Read the model definition and answer for the solid it produces. Units are mm, in the model's axes. Face numbers are marked on the shaded views. A direction names the side the tool comes from. Round coordinates to 2 decimals unless told otherwise and drop trailing zeros. Loops run counter-clockwise (first coordinate to the right, second up) from the corner with the lowest first, then second, coordinate; pieces in that order, holes last. Notation, with made-up numbers: (42.5, 31) - (53.5, 31) arc R16 ccw to (53.5, 59) - close; hole circle Ø10 at (82, 72). An arc over 180 degrees is marked (long way). Use one line per item in the form item = value. Start each with the question number.
```python
from build123d import *

# Parameters (mm, degrees)
SKETCH_R     = 12
PAD_DEPTH    = 30
PAD001_DEPTH = 30


with BuildPart() as part:
    # Sketch → Pad (new body)
    with BuildSketch(Plane.XY):
        with BuildLine():
            Line((29.808627, -133.970841), (29.808627, -73.970841))
            Line((29.808627, -73.970841), (-30.191373, -73.970841))
            Line((-30.191373, -73.970841), (-30.191373, -133.970841))
            Line((-59.898036, -134.146891), (-30.191373, -133.970841))
            ThreePointArc((-79.943921, -113.552778), (-74.10502, -127.922494), (-59.898036, -134.146891))
            Line((-79.943921, 100.605318), (-79.943921, -113.552778))
            ThreePointArc((-59.685634, 120.863606), (-74.010406, 114.930091), (-79.943921, 100.605318))
            Line((60.081005, 120.863606), (-59.685634, 120.863606))
            ThreePointArc((80.068853, 100.875757), (74.214548, 115.009301), (60.081005, 120.863606))
            Line((80.068853, -113.591927), (80.068853, 100.875757))
            ThreePointArc((59.515305, -134.144193), (74.048781, -128.125027), (80.068853, -113.591927))
            Line((29.808627, -133.970841), (59.515305, -134.144193))
        make_face()
        with Locations((0.120778, 29.919195)):
            Circle(SKETCH_R, mode=Mode.SUBTRACT)
        with Locations((-53.325886, -24.171413)):
            Circle(SKETCH_R, mode=Mode.SUBTRACT)
        with Locations((55.271923, 86.295181)):
            Circle(SKETCH_R, mode=Mode.SUBTRACT)
    extrude(amount=PAD_DEPTH)

    # Sketch → Pad001 (join)
    with BuildSketch(Plane.XY):
        with BuildLine():
            Line((29.808627, -133.970841), (29.808627, -73.970841))
            Line((29.808627, -73.970841), (-30.191373, -73.970841))
            Line((-30.191373, -73.970841), (-30.191373, -133.970841))
            Line((-59.898036, -134.146891), (-30.191373, -133.970841))
            ThreePointArc((-79.943921, -113.552778), (-74.10502, -127.922494), (-59.898036, -134.146891))
            Line((-79.943921, 100.605318), (-79.943921, -113.552778))
            ThreePointArc((-59.685634, 120.863606), (-74.010406, 114.930091), (-79.943921, 100.605318))
            Line((60.081005, 120.863606), (-59.685634, 120.863606))
            ThreePointArc((80.068853, 100.875757), (74.214548, 115.009301), (60.081005, 120.863606))
            Line((80.068853, -113.591927), (80.068853, 100.875757))
            ThreePointArc((59.515305, -134.144193), (74.048781, -128.125027), (80.068853, -113.591927))
            Line((29.808627, -133.970841), (59.515305, -134.144193))
        make_face()
        with Locations((0.120778, 29.919195)):
            Circle(SKETCH_R, mode=Mode.SUBTRACT)
        with Locations((-53.325886, -24.171413)):
            Circle(SKETCH_R, mode=Mode.SUBTRACT)
        with Locations((55.271923, 86.295181)):
            Circle(SKETCH_R, mode=Mode.SUBTRACT)
    extrude(amount=PAD001_DEPTH)


solid = part.part
```
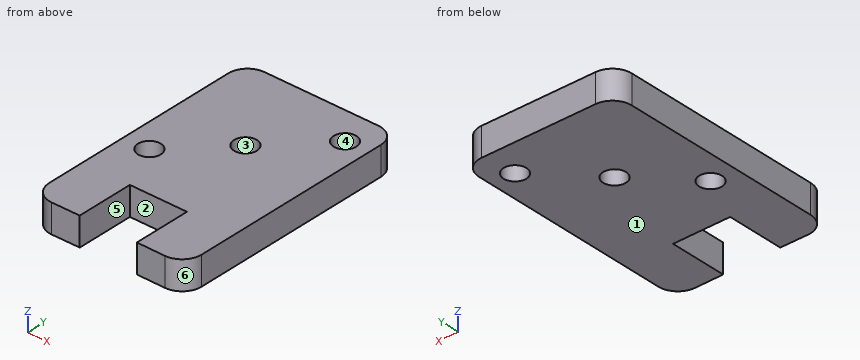
1) Flat-ended cylindrical pins translate along their axes: pin 1 (21.5 mm diameter, centred on x = 0.12, y = 29.92, fed in from -Z); pin 2 (8 mm diameter, centred on x = 51, z = 8.5, fed in from -Y). Find the tip coordinate at first contact, or state that the pin passes through.
2) A cutting plane is placed at B-B on x = 52. Write down the section's boundary in (y, z).
3) A cutting plane is placed at A-A on y = -109. Write down the section's boundary in (x, z).
4) Determine the mould class of the marked faces 1, 2, 3 and 4 for opening direction Y: +Y half, -Y half, draft (parallel to the pull), parting line (faces both ways), or undercut.
5) A cutting plane is placed at C-C on z = 22.5. Write down the section's boundary in (x, y), plus the area to 3 significant figures.
6) A cutting plane is placed at D-D on x = 20. Write down the section's boundary in (y, z), plus the area to 3 significant figures.
7) Straight lines are drawn through the part: line 1 (X direction, y = -95.5, z = 3); line 2 (Y direction, x = -36.5, z = 20.25); line 3 (X direction, y = 95, z = 22.5). For each, find the intervals that lie inside material, in ascending order. Write a range as from..to.
8) For the marked faces 5 and 6, determine the directions among +Z, -Z, +X, -X, +Y, -Y from which every point of the face is accessible in a straight line to the end or side of a thin tool.
Checks:
q1.pin_1 = through
q1.pin_2 = -134.12
q2.outline = (-134.1, 0) - (74.75, 0) - (74.75, 30) - (-134.1, 30) - close; (97.84, 0) - (120.86, 0) - (120.86, 30) - (97.84, 30) - close
q3.outline = (-79.94, 0) - (-30.19, 0) - (-30.19, 30) - (-79.94, 30) - close; (29.81, 0) - (80.07, 0) - (80.07, 30) - (29.81, 30) - close
q4.face_1 = draft
q4.face_2 = -Y half
q4.face_3 = undercut
q4.face_4 = undercut
q5.outline = (-79.94, -113.55) arc R20.6 ccw to (-59.9, -134.15) - (-30.19, -133.97) - (-30.19, -73.97) - (29.81, -73.97) - (29.81, -133.97) - (59.52, -134.14) arc R20.55 ccw to (80.07, -113.59) - (80.07, 100.88) arc R19.99 ccw to (60.08, 120.86) - (-59.69, 120.86) arc R20.26 ccw to (-79.94, 100.61) - close; hole circle Ø24 at (-53.33, -24.17); hole circle Ø24 at (0.12, 29.92); hole circle Ø24 at (55.27, 86.3)
q5.area = 35,500 mm²
q6.outline = (-73.97, 0) - (120.86, 0) - (120.86, 30) - (-73.97, 30) - close
q6.area = 5,850 mm²
q7.line_1 = -79.94..-30.19, 29.81..80.07
q7.line_2 = -134.01..120.86
q7.line_3 = -79.94..47.01, 63.53..80.07
q8.face_5 = +Z, -Z, -Y
q8.face_6 = +Z, -Z, +X, -Y
